from build123d import *

# Parameters (mm, degrees)
BOSS_EXTRUDE1_DEPTH = 46.101
SKETCH2_R           = 2.0193
CUT_EXTRUDE1_DEPTH  = 48.038886732


with BuildPart() as part:
    # Sketch1 → Boss-Extrude1 (new body)
    with BuildSketch(Plane.XY):
        with BuildLine():
            Line((-0.93173274, 6.79441227), (-5.41826726, 4.204110358))
            ThreePointArc((-5.41826726, 4.204110358), (-5.939202219, 3.429), (-6.35, 2.590301913))
            Line((-6.35, 2.590301913), (-6.35, -2.590301913))
            ThreePointArc((-6.35, -2.590301913), (-5.939202219, -3.429), (-5.41826726, -4.204110358))
            Line((-5.41826726, -4.204110358), (-0.93173274, -6.79441227))
            ThreePointArc((-0.93173274, -6.79441227), (0, -6.858), (0.93173274, -6.79441227))
            Line((0.93173274, -6.79441227), (5.41826726, -4.204110358))
            ThreePointArc((5.41826726, -4.204110358), (5.939202219, -3.429), (6.35, -2.590301913))
            Line((6.35, -2.590301913), (6.35, 2.590301913))
            ThreePointArc((6.35, 2.590301913), (5.939202219, 3.429), (5.41826726, 4.204110358))
            Line((5.41826726, 4.204110358), (0.93173274, 6.79441227))
            ThreePointArc((0.93173274, 6.79441227), (0, 6.858), (-0.93173274, 6.79441227))
        make_face()
    extrude(amount=BOSS_EXTRUDE1_DEPTH)

    # Sketch2 → Cut-Extrude1 (cut, through all)
    with BuildSketch(Plane.XY.offset(46.101)):
        Circle(SKETCH2_R)
    extrude(amount=-CUT_EXTRUDE1_DEPTH, mode=Mode.SUBTRACT)


solid = part.part
Design review of the part built by this model. Coordinates are the model's own, in mm. Give positions to 0.01 mm unless a question says otherwise; leave off trailing zeros. Write each loop counter-clockwise with the first axis right and the second up, starting at its lowest first coordinate (ties: lowest second). Pieces come first, ordered by that corner, then holes. Notation, with made-up numbers: M -5.75,60 L 40.25,60 A12 cw 40.25,75 Z; hole C 46.5,-36 d7. An arc over 180 degrees is marked long. Return JSON: item names as keys, results as strings. Group by question number.
Item 1: Take a section at B-B (x = 0). Give the boundary of the cut face in (y, z).
Item 2: Take a section at A-A (y = 0). Give the boundary of the cut face in (x, z), plus the area to 3 significant figures.
Item 3: Wall thickness on line 1 along Y through (x, z) = (0, 32); line 2 along X through (y, z) = (-0.75, 33); line 3 along Y through (x, z) = (-0.5, 31): over which ranges is each line inside the solid? List them lowest first.
Item 4: Clearance check with flat-ended pins moving along their axes: pin 1 Ø1 at (x, z) = (4, 7) entering from -Y; pin 2 Ø3 at (x, z) = (3.5, 27) entering from +Y; pin 3 Ø3.5 at (x, y) = (0, 0) entering from +Z. State where each tip first meets the part, or that it passes through.
Item 5: The part is to be moulded in two halves that separate along X. For faces 1 (the flat face through (3.21, 5.48, 22.73)), 2 (the cylindrical face through (-5.933, 3.44, 22.728)), 3 (the cylindrical face through (1.926, 0.607, 23.373)), say which applies: pulls with the +X half, pulls with the -X half, needs draft (parallel to the pull), parting line crosses it, or undercut.
Item 6: Take a section at C-C (z = 26.5). Give the boundary of the cut face in (x, y), plus the area to 3 significant figures.
Item 7: Take a section at D-D (y = -5.5). Give the boundary of the cut face in (x, z), plus the area to 3 significant figures.
Return value:
{
 "1": {"outline": "M -6.86,0 L -2.02,0 L -2.02,46.1 L -6.86,46.1 Z; M 2.02,0 L 6.86,0 L 6.86,46.1 L 2.02,46.1 Z"},
 "2": {"outline": "M -6.35,0 L -2.02,0 L -2.02,46.1 L -6.35,46.1 Z; M 2.02,0 L 6.35,0 L 6.35,46.1 L 2.02,46.1 Z", "area": "399 mm2"},
 "3": {"line 1": "y = -6.86 to -2.02, 2.02 to 6.86", "line 2": "x = -6.35 to -1.87, 1.87 to 6.35", "line 3": "y = -6.84 to -1.96, 1.96 to 6.84"},
 "4": {"pin 1": "stops at y = -5.31", "pin 2": "stops at y = 6.18", "pin 3": "passes through"},
 "5": {"face 1": "pulls with the +X half", "face 2": "pulls with the -X half", "face 3": "undercut"},
 "6": {"outline": "M -6.35,-2.59 A6.86 ccw -5.42,-4.2 L -0.93,-6.79 A6.86 ccw 0.93,-6.79 L 5.42,-4.2 A6.86 ccw 6.35,-2.59 L 6.35,2.59 A6.86 ccw 5.42,4.2 L 0.93,6.79 A6.86 ccw -0.93,6.79 L -5.42,4.2 A6.86 ccw -6.35,2.59 Z; hole C 0,0 d4.04", "area": "124 mm2"},
 "7": {"outline": "M -3.17,0 L 3.17,0 L 3.17,46.1 L -3.17,46.1 Z", "area": "293 mm2"}
}
